The listing builds one solid part. Answer for the finished solid, in the listing's coordinates (mm). Face numbers are marked on the shaded views. A direction names the side the tool comes from. Round coordinates to 2 decimals unless told otherwise and drop trailing zeros. Loops run counter-clockwise (first coordinate to the right, second up) from the corner with the lowest first, then second, coordinate; pieces in that order, holes last. Notation, with made-up numbers: (52, -29) -> (64, -29) arc R23 ccw to (64, -14) -> close; hole circle Ø2 at (-22.75, 63). An arc over 180 degrees is marked (long way). Use a Markdown table: item, result. Add a question column.
Q1. Consider line 1 (Z direction, x = 11.75, y = 21.5); line 2 (Y direction, x = 6, z = 0); line 3 (Y direction, x = 4, z = 4.5). Determine where each line is inside the solid, lowest interval first.
Q2. Which of the six approach directions +Z, -Z, +X, -X, +Y, -Y give full straight-line access (tool end or side, diameter ignored) to the marked faces 1, 2, 3, 4 and 5?
Q3. Section A-A on z = 0 is taken. Give the vertices of the cut face in (x, y).
Q4. Given pin 1 Ø9.5 at (x, y) = (7.5, 6) entering from +Z; pin 2 Ø3 at (x, y) = (9, 21.5) entering from -Z; pin 3 Ø7.5 at (x, y) = (10, 17) entering from +Z, each flat-ended and moving along its own axis, determine where each tip first touches the part or whether it passes through.
Q5. Section B-B on x = 13.25 is taken. Give the vertices of the cut face in (y, z).
Q6. For a pull along Z with two mould halves and no side action, classify the marked faces 6, 7 and 8 as released by +Z, released by -Z, zero draft, split by the parting line, or undercut.
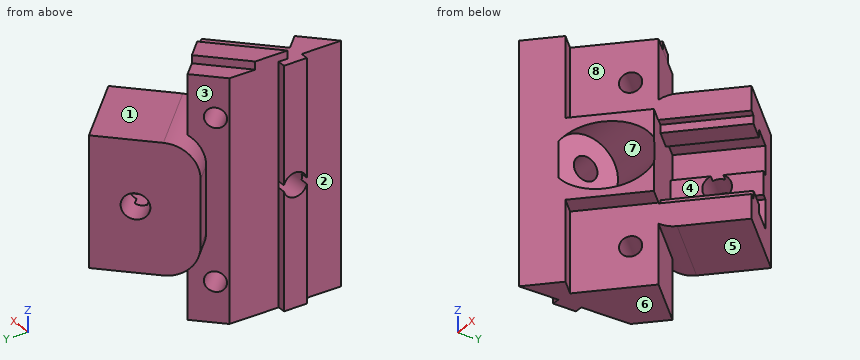
from build123d import *

# Parameters (mm, degrees)
MAIN_EXTRUSION_DEPTH                   = 15
ESQUISSE2_W                            = 10
ESQUISSE2_H                            = 9.5
WINDOW_EXTRUSION_DEPTH                 = 2.5
ESQUISSE5_R                            = 1.25
WINDOW_HOLE_EXTRUSION_DEPTH            = 11.457106781
FIXATION_TOP_MAKERBEAM_EXTRUSION_DEPTH = 10
ESQUISSE3_R                            = 1.5
WINDOW_HOLE_FIXATION_DEPTH             = 17.556349186
ESQUISSE4_R                            = 4.1
CENTRAL_FIXATION_DEPTH                 = 13.556349186
BOSS_EXTRU_2_DEPTH                     = 1
BOSS_EXTRU_6_DEPTH                     = 12
CONG_1_R                               = 4
ESQUISSE11_R                           = 1.6
ENL_V_MAT_EXTRU_2_DEPTH                = 25


with BuildPart() as part:
    # Esquisse1 → Main Extrusion (new body, symmetric)
    with BuildSketch(Plane.XY):
        Polygon((0, 0), (0, 5), (-1, 5), (-1, 7.9), (0, 7.9), (0, 14.142135624), (3.181980515, 17.324116139), (10.253048327, 10.253048327), align=None)
    extrude(amount=MAIN_EXTRUSION_DEPTH, both=True)

    # Esquisse2 → Window Extrusion (cut)
    with BuildSketch(Plane(origin=(0, 0, 0), x_dir=(0, 0, -1), z_dir=(0.707106781, -0.707106781, 0))):
        with Locations((10, 9.75)):
            Rectangle(ESQUISSE2_W, ESQUISSE2_H)
    window_extrusion = extrude(amount=-WINDOW_EXTRUSION_DEPTH, mode=Mode.SUBTRACT)

    # Esquisse5 → Window Hole Extrusion (cut, through all)
    with BuildSketch(Plane(origin=(-1.767766953, 1.767766953, 0), x_dir=(0, 0, -1), z_dir=(0.707106781, -0.707106781, 0))):
        with Locations((10, 11.5)):
            Circle(ESQUISSE5_R)
    window_hole_extrusion = extrude(amount=-WINDOW_HOLE_EXTRUSION_DEPTH, mode=Mode.SUBTRACT)

    # Esquisse7 → Fixation Top MakerBeam Extrusion (add)
    with BuildSketch(Plane(origin=(10.253048327, 10.253048327, 0), x_dir=(0, 0, -1), z_dir=(0.707106781, 0.707106781, 0))):
        Polygon((-5.1, 2.5), (-5.1, 3.55), (-4.1, 3.55), (-4.1, 6.45), (-5.1, 6.45), (-5.1, 10), (-8.1, 10), (-8.1, 2.5), align=None)
    fixation_top_makerbeam_extrusion = extrude(amount=FIXATION_TOP_MAKERBEAM_EXTRUSION_DEPTH)

    # Window Symetry: Window Extrusion, Window Hole Extrusion, Fixation Top MakerBeam Extrusion across plane
    add(window_extrusion.mirror(Plane.XY), mode=Mode.SUBTRACT)
    add(window_hole_extrusion.mirror(Plane.XY), mode=Mode.SUBTRACT)
    add(fixation_top_makerbeam_extrusion.mirror(Plane.XY))

    # Esquisse3 → Window Hole Fixation (cut, through all)
    with BuildSketch(Plane.ZY.offset(1)):
        with Locations((0, 6.45)):
            Circle(ESQUISSE3_R)
    extrude(amount=-WINDOW_HOLE_FIXATION_DEPTH, mode=Mode.SUBTRACT)

    # Esquisse4 → Central Fixation (cut, through all)
    with BuildSketch(Plane.ZY.offset(-3)):
        with Locations((0, 6.45)):
            Circle(ESQUISSE4_R)
    extrude(amount=-CENTRAL_FIXATION_DEPTH, mode=Mode.SUBTRACT)

    # Esquisse6 → Boss.-Extru.2 (add)
    with BuildSketch(Plane.XY.offset(15)):
        Polygon((0, 10.88944443), (4.808326112, 15.697770542), (6.858935778, 13.647160877), (0, 6.788225099), align=None)
    extrude(amount=BOSS_EXTRU_2_DEPTH)

    # Esquisse8 → Boss.-Extru.6 (add)
    with BuildSketch(Plane(origin=(17.324116139, 17.324116139, 0), x_dir=(0, 0, -1), z_dir=(0.707106781, 0.707106781, 0))):
        Polygon((-8.1, 10), (-1.45, 10), (-1.45, 9), (1.45, 9), (1.45, 10), (8.1, 10), (8.1, 13), (-8.1, 13), align=None)
    extrude(amount=-BOSS_EXTRU_6_DEPTH)

    # Congé1
    cong_1_edges = [part.edges().sort_by_distance(p)[0] for p in [
        (0.707106781, 16.970562748, -8.1),
        (0.707106781, 16.970562748, 8.1),
    ]]
    fillet(cong_1_edges, radius=CONG_1_R)

    # Esquisse11 → Enlèv. mat.-Extru.2 (cut, through all)
    with BuildSketch(Plane(origin=(-9.192388155, 9.192388155, 0), x_dir=(0, 0, 1), z_dir=(-0.707106781, 0.707106781, 0))):
        with Locations((0, 19.5)):
            Circle(ESQUISSE11_R)
    extrude(amount=-ENL_V_MAT_EXTRU_2_DEPTH, mode=Mode.SUBTRACT)


solid = part.part
Checked values:
| question | item | result |
|---|---|---|
| 1 | line 1 | z = -8.1 to -5.1, 5.1 to 8.1 |
| 1 | line 2 | y = 10.55 to 14.51, 18.73 to 19.31, 23.84 to 24.38 |
| 1 | line 3 | y = 4 to 16.51, 18.14 to 22.38 |
| 2 | face 1 | +Z, +X, +Y |
| 2 | face 2 | +Z, -Z, -X, -Y |
| 2 | face 3 | -X |
| 2 | face 4 | +X |
| 2 | face 5 | -Z, +X, +Y |
| 3 | outline | (-0.35, 18.03) -> (1.77, 15.91) -> (0, 14.14) -> (0, 7.95) -> (3, 7.95) -> (3, 10.55) -> (9.96, 10.55) -> (3.89, 16.62) -> (6.29, 19.02) -> (3.46, 21.85) -> close; (0, 0) -> (3, 3) -> (3, 4.95) -> (0, 4.95) -> close; (5.73, 24.11) -> (8.56, 21.28) -> (10.96, 23.69) -> (8.13, 26.52) -> close |
| 4 | pin 1 | stops at z = 15 |
| 4 | pin 2 | stops at z = -8.1 |
| 4 | pin 3 | stops at z = 8.1 |
| 5 | outline | (16.79, -8.1) -> (21.4, -8.1) -> (21.4, -4.1) -> (18.27, -4.1) -> (18.27, -5.1) -> (16.79, -5.1) -> close; (16.79, 5.1) -> (18.27, 5.1) -> (18.27, 4.1) -> (21.4, 4.1) -> (21.4, 8.1) -> (16.79, 8.1) -> close |
| 6 | face 6 | released by -Z |
| 6 | face 7 | undercut |
| 6 | face 8 | zero draft |
